```python
from build123d import *

# Parameters (mm, degrees)
F1_DEPTH = 30
F2_W     = 11
F2_H     = 15
F3_DEPTH = 11
F4_W     = 15
F4_H     = 8
F5_DEPTH = 11
F6_ANGLE = -90
F8_DEPTH = 11


with BuildPart() as f1:
    # F0 (on Front) → F1 (new body)
    with BuildSketch(Plane.XZ):
        Polygon((0, 30), (0, 0), (40, 0), (40, 11), (11, 11), (11, 30), align=None)
    extrude(amount=F1_DEPTH)

    # F2 (on face) → F3 (cut, through all)
    with BuildSketch(Plane.XY.offset(11)):
        with Locations((34.5, -22.5)):
            Rectangle(F2_W, F2_H)
    extrude(amount=-F3_DEPTH, mode=Mode.SUBTRACT)

    # F4 (on face) → F5 (cut, through all)
    with BuildSketch(Plane.YZ.offset(11)):
        with Locations((-22.5, 26)):
            Rectangle(F4_W, F4_H)
    extrude(amount=-F5_DEPTH, mode=Mode.SUBTRACT)


with BuildPart() as f1_1:
    # F6: moved
    add(f1.part.rotate(Axis((0, 0, 15), (0, 0, 1)), F6_ANGLE))

    # F7 (on face) → F8 (join, through all)
    with BuildSketch(Plane.XZ.offset(11)):
        Polygon((-15, 22), (-15, 30), (-30, 22), align=None)
    extrude(amount=-F8_DEPTH)


solid = f1_1.part
```
Check sheet for the modelled part. Datum: model origin and axes. Units: mm. A direction names the side the tool comes from. Give positions to 0.01 mm unless a question says otherwise; leave off trailing zeros. Order: outer loops, then holes, each group sorted by start corner. A loop starts at its lowest first (then second) coordinate and runs counter-clockwise, first axis right, second up. Notation, with made-up numbers: M -20,-5.5 L -2,-5.5 A24 cw -2,5.5 Z; hole C -24,-18 d11. An arc over 180 degrees is marked long. Answer in a Markdown table with one row per item.
1) Cross-section at A-A, the plane x = -8. Enter the section's corners in (y, z).
Filled sheet:
| item | result |
|---|---|
| outline | M -40,0 L 0,0 L 0,30 L -11,30 L -11,11 L -40,11 Z |
2) Cross-section at D-D, the plane y = -8. Enter the section's corners in (x, z), plus the area to 3 significant figures.
Filled sheet:
| item | result |
|---|---|
| outline | M -30,0 L 0,0 L 0,30 L -15,30 L -30,22 Z |
| area | 840 mm2 |
3) Access from +Z, -Z, +X, -X, +Y, -Y to the whole of each face (thin tool, end or side, straight path). Record for faces 1 (the flat face through (-7, -6, 30)), 2 (the flat face through (-15, -11, 21)), 3 (the flat face through (-23, -29, 6)).
Filled sheet:
| item | result |
|---|---|
| face 1 | +Z, +X, -X, +Y, -Y |
| face 2 | +Z, +X, -X, -Y |
| face 3 | +Z, -Z, -X, -Y |
4) Cross-section at C-C, the plane y = -33. Enter the section's corners in (x, z).
Filled sheet:
| item | result |
|---|---|
| outline | M -15,0 L 0,0 L 0,11 L -15,11 Z |
5) Gauge pin test, flat ends, axial feed: P1, Ø3.5, axis at x = -23.5, z = 6.5, coming from the -Y side; P2, Ø8.5, axis at x = -18, y = -20.5, coming from the +Z side; P3, Ø4, axis at y = -7.5, z = 25.5, coming from the -X side. Record the tip position at first contact, or that the pin passes through.
Filled sheet:
| item | result |
|---|---|
| P1 | stops at y = -29 |
| P2 | stops at z = 11 |
| P3 | stops at x = -27.19 |
6) Cross-section at B-B, the plane z = 2.25. Enter the section's corners in (x, y).
Filled sheet:
| item | result |
|---|---|
| outline | M -30,-29 L -15,-29 L -15,-40 L 0,-40 L 0,0 L -30,0 Z |
7) Thickness scan on L1, parallel to X at y = -33, z = 1.5; L2, parallel to Z at x = -18, y = -23.5; L3, parallel to Y at x = -8, z = 16.5. Record the ranges inside material, lowest first. Write a range as [from, to].
Filled sheet:
| item | result |
|---|---|
| L1 | x = [-15, 0] |
| L2 | z = [0, 11] |
| L3 | y = [-11, 0] |
